Here's how the part is built. I have some questions about the finished solid (model axes, mm). A direction names the side the tool comes from. Coordinates: 2 decimals unless noted, no trailing zeros. Write each loop counter-clockwise with the first axis right and the second up, starting at its lowest first coordinate (ties: lowest second). Pieces come first, ordered by that corner, then holes.
Item 1: If I drill on line 1 (Y direction, x = 86, z = 4.35); line 2 (X direction, y = 86, z = 3.6); line 3 (X direction, y = 31.5, z = 4.3), over which ranges is the centre line in solid material (lowest first)?
Item 2: For faces 1 (the face through (64.01, 131.79, 2.46)), 2 (the face through (73.534, 179.825, 2.465)), which set-ups out of +Z, -Z, +X, -X, +Y, -Y let a thin tool reach every point of the face, with its end or its side?
Item 3: If we section it at D-D (x = 16): Please give me the cut outline in (y, z).
Item 4: We'd pull the mould along Y, two halves only. Please class faces 3 (the face through (61.735, 87.89, 2.465)), 4 (the face through (62.16, 159.37, 2.46)), 5 (the face through (13.486, 101.008, 2.465)): +Y half, -Y half, draft (parallel to the pull), parting line (faces both ways), or undercut.
Item 5: If we section it at B-B (x = 84): Please give me the cut outline in (y, z), then the cut area to 3 significant figures.
Item 6: I'm going to push flat-ended pins straight in: pin 1 Ø6.5 at (x, y) = (26.37, 31.38) entering from +Z; pin 2 Ø1 at (y, z) = (52.5, 3) entering from +X; pin 3 Ø3 at (y, z) = (151.5, 3) entering from +X. Where does each tip first touch, or does it pass through?
Item 7: If we section it at A-A (y = 103): Please give me the cut outline in (x, z).
Item 8: If we section it at C-C (y = 135): Please give me the cut outline in (x, z).
from build123d import *

# Parameters (mm, degrees)
SKETCH_R     = 2.5
PAD_DEPTH    = 5
CHAMFER_SIZE = 2


with BuildPart() as part:
    # Sketch → Pad (new body)
    with BuildSketch(Plane.XY):
        with BuildLine():
            ThreePointArc((51.58022, 192.5), (13.118557, 99.645332), (0, 0))
            Line((50, 0), (0, 0))
            ThreePointArc((94.88149, 167.5), (61.414848, 86.70438), (50, 0))
            Line((94.88149, 167.5), (51.58022, 192.5))
        make_face()
        with Locations((26.369909, 31.376067)):
            Circle(SKETCH_R, mode=Mode.SUBTRACT)
        with Locations((58.729197, 152.142574)):
            Circle(SKETCH_R, mode=Mode.SUBTRACT)
        with Locations((37.266703, 93.174856)):
            Circle(SKETCH_R, mode=Mode.SUBTRACT)
        with BuildLine():
            ThreePointArc((52.678296, 188.401924), (51.150584, 185.681361), (49.645145, 182.948411))
            Line((57.959305, 160.105442), (49.645145, 182.948411))
            ThreePointArc((65.323984, 156.671236), (62.110143, 159.393037), (57.959305, 160.105442))
            Line((65.323984, 156.671236), (90.453773, 165.817731))
            ThreePointArc((90.783414, 166.401924), (90.618448, 166.109909), (90.453773, 165.817731))
            Line((90.783414, 166.401924), (52.678296, 188.401924))
        make_face(mode=Mode.SUBTRACT)
        with BuildLine():
            Line((47, 3), (3, 3))
            ThreePointArc((3.099971, 9.239456), (3.037245, 6.119932), (3, 3))
            Line((21.721729, 24.864967), (3.099971, 9.239456))
            ThreePointArc((21.721729, 24.864967), (25.672663, 23.40651), (29.816831, 24.156737))
            Line((29.816831, 24.156737), (47.006619, 3.670746))
            ThreePointArc((47.006619, 3.670746), (47.003143, 3.335375), (47, 3))
        make_face(mode=Mode.SUBTRACT)
        with BuildLine():
            ThreePointArc((19.858808, 36.024247), (18.400351, 32.073313), (19.150579, 27.929145))
            Line((19.150579, 27.929145), (3.267378, 14.601557))
            ThreePointArc((6.531221, 51.907447), (4.44189, 33.29452), (3.267378, 14.601557))
            Line((19.858808, 36.024247), (6.531221, 51.907447))
        make_face(mode=Mode.SUBTRACT)
        with BuildLine():
            Line((22.922986, 38.595397), (7.297475, 57.217156))
            ThreePointArc((10.506305, 75.415332), (8.791837, 66.335649), (7.297475, 57.217156))
            Line((31.558499, 87.569822), (10.506305, 75.415332))
            ThreePointArc((31.558499, 87.569822), (35.19615, 85.44745), (39.407635, 85.466652))
            Line((39.407635, 85.466652), (52.778916, 62.306914))
            ThreePointArc((52.778916, 62.306914), (52.121868, 58.695396), (51.50408, 55.076955))
            Line((31.018088, 37.887168), (51.50408, 55.076955))
            ThreePointArc((31.018088, 37.887168), (27.067155, 39.345625), (22.922986, 38.595397))
        make_face(mode=Mode.SUBTRACT)
        with BuildLine():
            Line((32.881009, 26.727888), (47.127329, 9.749785))
            ThreePointArc((50.567342, 49.06931), (48.272929, 29.459801), (47.127329, 9.749785))
            Line((33.589239, 34.82299), (50.567342, 49.06931))
            ThreePointArc((32.881009, 26.727888), (34.339466, 30.678821), (33.589239, 34.82299))
        make_face(mode=Mode.SUBTRACT)
        with BuildLine():
            ThreePointArc((54.200535, 158.737362), (51.478734, 155.52352), (50.766329, 151.372683))
            Line((50.766329, 151.372683), (31.282699, 144.281222))
            ThreePointArc((47.109074, 178.220991), (38.779749, 161.445154), (31.282699, 144.281222))
            Line((54.200535, 158.737362), (47.109074, 178.220991))
        make_face(mode=Mode.SUBTRACT)
        with BuildLine():
            Line((52.134409, 147.613912), (29.291441, 139.299752))
            ThreePointArc((29.291441, 139.299752), (26.026349, 130.655724), (22.97128, 121.935254))
            Line((35.12577, 100.88306), (22.97128, 121.935254))
            ThreePointArc((42.974906, 98.77989), (39.337255, 100.902263), (35.12577, 100.88306))
            Line((42.974906, 98.77989), (66.134645, 112.151172))
            ThreePointArc((68.645583, 119.049918), (67.371384, 115.607362), (66.134645, 112.151172))
            Line((59.499088, 144.179706), (68.645583, 119.049918))
            ThreePointArc((52.134409, 147.613912), (55.348251, 144.892112), (59.499088, 144.179706))
        make_face(mode=Mode.SUBTRACT)
        with BuildLine():
            Line((63.257859, 145.547787), (70.838167, 124.72106))
            ThreePointArc((87.518791, 160.492774), (78.655902, 142.850599), (70.838167, 124.72106))
            Line((66.692065, 152.912466), (87.518791, 160.492774))
            ThreePointArc((63.257859, 145.547787), (65.979659, 148.761628), (66.692065, 152.912466))
        make_face(mode=Mode.SUBTRACT)
        with BuildLine():
            Line((42.871737, 87.466652), (53.953407, 68.272637))
            ThreePointArc((64.168922, 106.397459), (58.504211, 87.484283), (53.953407, 68.272637))
            Line((44.974906, 95.315789), (64.168922, 106.397459))
            ThreePointArc((42.871737, 87.466652), (44.994109, 91.104304), (44.974906, 95.315789))
        make_face(mode=Mode.SUBTRACT)
        with BuildLine():
            Line((29.558499, 91.033924), (11.602288, 80.666901))
            ThreePointArc((21.294646, 116.83927), (16.004956, 98.871924), (11.602288, 80.666901))
            Line((31.661668, 98.88306), (21.294646, 116.83927))
            ThreePointArc((31.661668, 98.88306), (29.539296, 95.245409), (29.558499, 91.033924))
        make_face(mode=Mode.SUBTRACT)
    extrude(amount=PAD_DEPTH)

    # Chamfer
    chamfer_edges = [part.edges().sort_by_distance(p)[0] for p in [
        (23.869909, 31.376067, 5),
        (34.766703, 93.174856, 5),
        (56.229197, 152.142574, 5),
    ]]
    chamfer(chamfer_edges, length=CHAMFER_SIZE)


solid = part.part
Answer list:
1. line 1: y = 151.08 to 157.65, 159.94 to 164.2, 169.16 to 172.63
1. line 2: x = 9.73 to 12.79, 20.84 to 28.84, 33.73 to 43.72, 58.11 to 61.23
1. line 3: x = 1.29 to 4.29, 18.37 to 22.57, 30.17 to 34.37, 48.46 to 51.48
2. face 1: +Z, -Z
2. face 2: +Z, -Z, +X, +Y
3. outline: (0, 0) - (3, 0) - (3, 5) - (0, 5) - close; (20.06, 0) - (25.29, 0) - (25.29, 5) - (20.06, 5) - close; (40.62, 0) - (46.85, 0) - (46.85, 5) - (40.62, 5) - close; (78.59, 0) - (83.21, 0) - (83.21, 5) - (78.59, 5) - close; (98.85, 0) - (109.84, 0) - (109.84, 5) - (98.85, 5) - close
4. face 3: -Y half
4. face 4: undercut
4. face 5: +Y half
5. outline: (147.05, 0) - (153.79, 0) - (153.79, 5) - (147.05, 5) - close; (159.21, 0) - (163.47, 0) - (163.47, 5) - (159.21, 5) - close; (170.32, 0) - (173.78, 0) - (173.78, 5) - (170.32, 5) - close
5. area: 72.3 mm2
6. pin 1: stops at z = 3.75
6. pin 2: stops at x = 54.22
6. pin 3: stops at x = 86.98
7. outline: (14.03, 0) - (17.14, 0) - (17.14, 5) - (14.03, 5) - close; (29.28, 0) - (33.9, 0) - (33.9, 5) - (29.28, 5) - close; (50.28, 0) - (58.28, 0) - (58.28, 5) - (50.28, 5) - close; (63.06, 0) - (66.23, 0) - (66.23, 5) - (63.06, 5) - close
8. outline: (24.44, 0) - (27.64, 0) - (27.64, 5) - (24.44, 5) - close; (62.84, 0) - (67.1, 0) - (67.1, 5) - (62.84, 5) - close; (75.12, 0) - (78.41, 0) - (78.41, 5) - (75.12, 5) - close
